Check sheet for the drawn part. Datum: minimum x, y, z corner. Units: mm. Give positions to 0.01 mm unless a question says otherwise; leave off trailing zeros. Write each loop counter-clockwise with the first axis right and the second up, starting at its lowest first coordinate (ties: lowest second). Pieces come first, ordered by that corner, then holes. Notation, with made-up numbers: (85.25, -9.5) -> (94.25, -9.5) arc R23 cw to (94.25, 2.5) -> close; hole circle Ø3 at (8, 74.25). An arc over 180 degrees is marked (long way). Write item = value, one per line. Start each with the question number.
1. Thickness scan on line 1 along Z through (x, y) = (34, 0.9); line 2 along X through (y, z) = (2.7, 6). Record the ranges inside material, lowest first.
2. Cross-section at B-B, the plane x = 27.4. Record the cut outline in (y, z).
3. Cross-section at D-D, the plane y = 1.7. State how many separate pieces and enclosed holes the cut face has, plus the area to 3 significant figures.
4. Cross-section at C-C, the plane x = 38.1. Record the cut outline in (y, z).
5. Cross-section at A-A, the plane z = 16.7. Record the cut outline in (x, y).
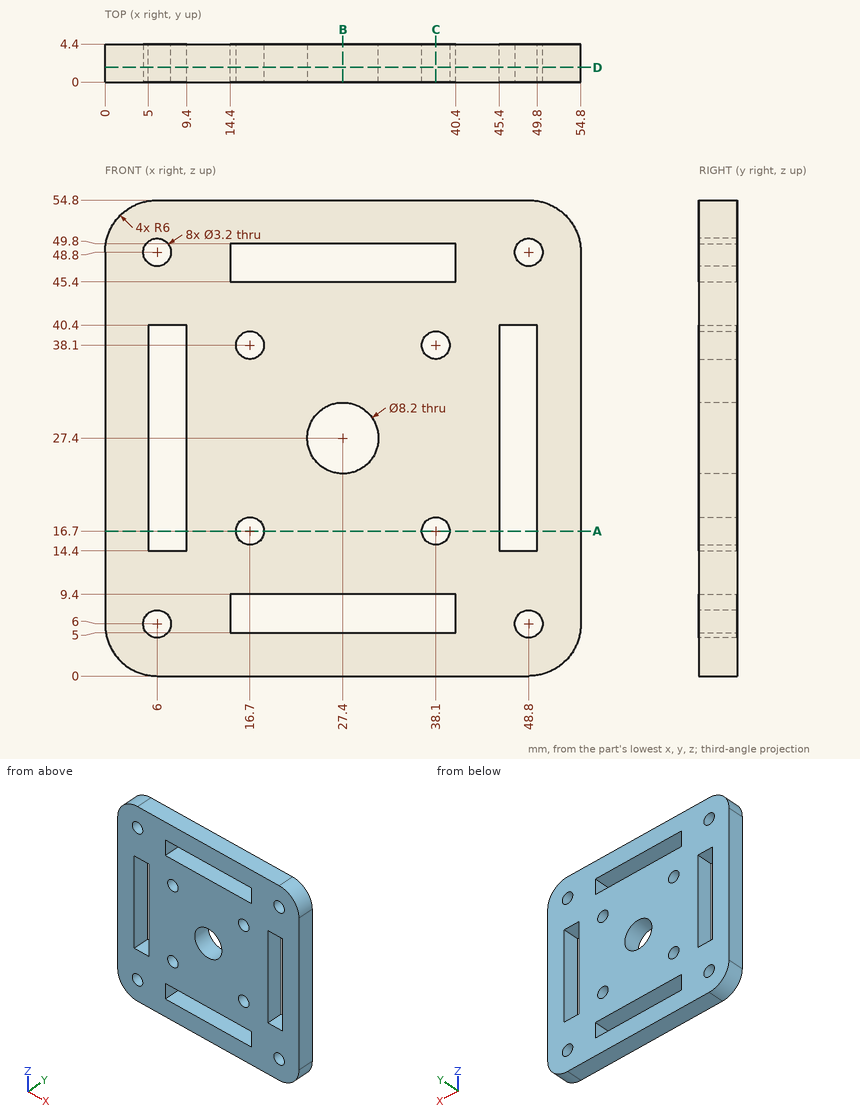
Answers:
q1.line_1 = 0 to 5, 9.4 to 45.4, 49.8 to 54.8
q1.line_2 = 0 to 4.4, 7.6 to 14.4, 40.4 to 47.2, 50.4 to 54.8
q2.outline = (0, 0) -> (4.4, 0) -> (4.4, 5) -> (0, 5) -> close; (0, 9.4) -> (4.4, 9.4) -> (4.4, 23.3) -> (0, 23.3) -> close; (0, 31.5) -> (4.4, 31.5) -> (4.4, 45.4) -> (0, 45.4) -> close; (0, 49.8) -> (4.4, 49.8) -> (4.4, 54.8) -> (0, 54.8) -> close
q3.separate_pieces = 1
q3.enclosed_holes = 13
q3.area = 2,400 mm^2
q4.outline = (0, 0) -> (4.4, 0) -> (4.4, 5) -> (0, 5) -> close; (0, 9.4) -> (4.4, 9.4) -> (4.4, 15.1) -> (0, 15.1) -> close; (0, 18.3) -> (4.4, 18.3) -> (4.4, 36.5) -> (0, 36.5) -> close; (0, 39.7) -> (4.4, 39.7) -> (4.4, 45.4) -> (0, 45.4) -> close; (0, 49.8) -> (4.4, 49.8) -> (4.4, 54.8) -> (0, 54.8) -> close
q5.outline = (0, 0) -> (5, 0) -> (5, 4.4) -> (0, 4.4) -> close; (9.4, 0) -> (15.1, 0) -> (15.1, 4.4) -> (9.4, 4.4) -> close; (18.3, 0) -> (36.5, 0) -> (36.5, 4.4) -> (18.3, 4.4) -> close; (39.7, 0) -> (45.4, 0) -> (45.4, 4.4) -> (39.7, 4.4) -> close; (49.8, 0) -> (54.8, 0) -> (54.8, 4.4) -> (49.8, 4.4) -> close
